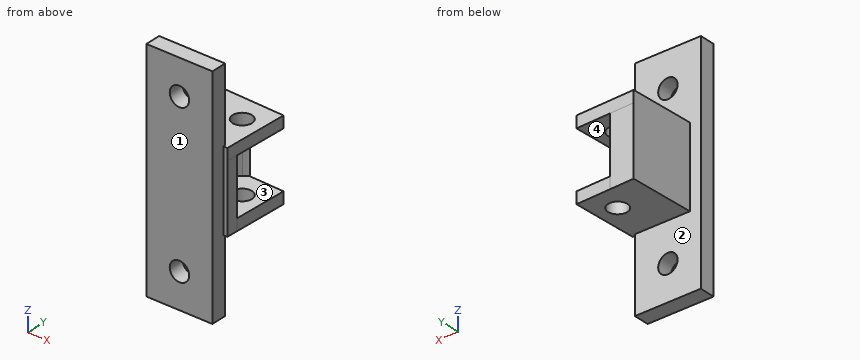
```python
from build123d import *

# Parameters (mm, degrees)
BOSS_EXTRUDE1_DEPTH = 22.352
BOSS_EXTRUDE3_START = -3.81
SKETCH2_R           = 3.175
BOSS_EXTRUDE3_DEPTH = 3.81
BOSS_EXTRUDE4_DEPTH = 3.81
CUT_EXTRUDE1_START  = -3.81
SKETCH6_R           = 3.175
CUT_EXTRUDE1_DEPTH  = 3.81
SKETCH7_W           = 21.59
SKETCH7_H           = 74.422
BOSS_EXTRUDE6_DEPTH = 5.08
SKETCH9_R           = 3.175
CUT_EXTRUDE2_DEPTH  = 6.35


with BuildPart() as part:
    # Sketch1 → Boss-Extrude1 (new body)
    with BuildSketch(Plane.XY):
        with BuildLine():
            ThreePointArc((-352.162161707, 117.383467749), (-351.384007065, 117.9545664), (-350.552048848, 118.44397813))
            Line((-350.552048848, 118.44397813), (-358.467972096, 118.728192663))
            Line((-358.467972096, 118.728192663), (-359.243555017, 97.126711503))
            Line((-359.243555017, 97.126711503), (-339.97264358, 96.434805718))
            Line((-339.97264358, 96.434805718), (-339.835936837, 100.242352338))
            Line((-339.835936837, 100.242352338), (-346.486451601, 100.481133449))
            ThreePointArc((-346.486451601, 100.481133449), (-349.816499797, 101.211177598), (-352.67617906, 103.067092457))
            ThreePointArc((-352.67617906, 103.067092457), (-355.663551295, 110.341766857), (-352.162161707, 117.383467749))
        make_face()
    extrude(amount=-BOSS_EXTRUDE1_DEPTH)

    # Sketch2 → Boss-Extrude3 (add)
    with BuildSketch(Plane(origin=(0, 0, -22.352), x_dir=(-1, 0, 0), z_dir=(0, 0, -1)).offset(BOSS_EXTRUDE3_START)):
        with BuildLine():
            ThreePointArc((346.486451601, 100.481133449), (355.434706729, 107.897354875), (350.552048848, 118.44397813))
            Line((350.552048848, 118.44397813), (339.197060659, 118.036286878))
            Line((339.197060659, 118.036286878), (339.835936837, 100.242352338))
            Line((339.835936837, 100.242352338), (346.486451601, 100.481133449))
        make_face()
        with Locations((346.144684744, 110)):
            Circle(SKETCH2_R, mode=Mode.SUBTRACT)
    extrude(amount=BOSS_EXTRUDE3_DEPTH)

    # Sketch3 → Boss-Extrude4 (add)
    with BuildSketch(Plane.XY):
        Polygon((-358.467972096, 118.728192663), (-359.243555017, 97.126711503), (-339.97264358, 96.434805718), (-339.197060659, 118.036286878), align=None)
    extrude(amount=BOSS_EXTRUDE4_DEPTH)

    # Sketch6 → Cut-Extrude1 (cut)
    with BuildSketch(Plane(origin=(0, 0, 0), x_dir=(-1, 0, 0), z_dir=(0, 0, -1)).offset(CUT_EXTRUDE1_START)):
        with Locations((346.144684744, 110)):
            Circle(SKETCH6_R)
    extrude(amount=CUT_EXTRUDE1_DEPTH, mode=Mode.SUBTRACT)

    # Sketch7 → Boss-Extrude6 (add)
    with BuildSketch(Plane(origin=(0, 97.126711503, 0), x_dir=(1, 0, 0), z_dir=(0, 1, 0))):
        with Locations((-352.044558269, 9.271)):
            Rectangle(SKETCH7_W, SKETCH7_H)
    extrude(amount=-BOSS_EXTRUDE6_DEPTH)

    # Sketch9 → Cut-Extrude2 (cut)
    with BuildSketch(Plane(origin=(0, 97.126711503, 0), x_dir=(1, 0, 0), z_dir=(0, 1, 0))):
        with Locations(Location((-352.044558269, -16.51, 0), (0, 0, 270))):
            Circle(SKETCH9_R)
        with Locations(Location((-352.044558269, 35.052, 0), (0, 0, 270))):
            Circle(SKETCH9_R)
    extrude(amount=-CUT_EXTRUDE2_DEPTH, mode=Mode.SUBTRACT)


solid = part.part
```
Build history of the part. All positions in model axes, mm. Face numbers are marked on the shaded views. Round coordinates to 2 decimals unless told otherwise and drop trailing zeros. Write each loop counter-clockwise with the first axis right and the second up, starting at its lowest first coordinate (ties: lowest second). Pieces come first, ordered by that corner, then holes. Notation, with made-up numbers: (53, -22.75) -> (109, -22.75) arc R21 ccw to (109, -3.75) -> close; hole circle Ø2 at (78, -18). An arc over 180 degrees is marked (long way). Put each result on its own line as item: value.
Item 1: Wall check: probe 1 along Z at (x, y) = (-350.5, 113.25); probe 2 along X at (y, z) = (94.2, 16.51); probe 3 along Y at (x, z) = (-358, 18.5). Give the ranges that are in metal, low to high. Write a range as from..to.
Here are the results:
probe 1: z = -22.35..-18.54, 0..3.81
probe 2: x = -362.84..-355.22, -348.87..-341.25
probe 3: y = 92.05..97.13
Item 2: Flat gauge pins, fed straight in: P1, Ø10, axis at x = -346.14, y = 110, coming from the +Z side; P2, Ø5, axis at x = -352.04, z = 16.51, coming from the -Y side; P3, Ø6, axis at x = -359, y = 109, coming from the -Z side; P4, Ø4, axis at x = -346, z = -17.5, coming from the +Y side. Where does each tip first touch, or does it go through?
Here are the results:
P1: stops at z = 3.81
P2: passes through
P3: stops at z = -22.35
P4: stops at y = 118.34
Item 3: Slice it at D-D, the plane y = 102. Give the cut face in (x, z), plus the area to 3 significant figures.
Here are the results:
outline: (-359.07, -22.35) -> (-339.77, -22.35) -> (-339.77, -18.54) -> (-351.31, -18.54) -> (-351.31, 0) -> (-339.77, 0) -> (-339.77, 3.81) -> (-359.07, 3.81) -> close
area: 291 mm^2
Item 4: Slice it at C-C, the plane y = 111. Give the cut face in (x, z).
Here are the results:
outline: (-358.75, -22.35) -> (-349.16, -22.35) -> (-349.16, -18.54) -> (-355.62, -18.54) -> (-355.62, 0) -> (-349.16, 0) -> (-349.16, 3.81) -> (-358.75, 3.81) -> close; (-343.13, -22.35) -> (-339.45, -22.35) -> (-339.45, -18.54) -> (-343.13, -18.54) -> close; (-343.13, 0) -> (-339.45, 0) -> (-339.45, 3.81) -> (-343.13, 3.81) -> close
Item 5: Slice it at A-A, the plane z = 2. Give the cut face in (x, y) (3 decimals).
Here are the results:
outline: (-362.84, 92.047) -> (-341.25, 92.047) -> (-341.25, 96.481) -> (-339.973, 96.435) -> (-339.197, 118.036) -> (-358.468, 118.728) -> (-359.244, 97.127) -> (-362.84, 97.127) -> close; hole circle Ø6.35 at (-346.145, 110)
Item 6: Two-plate mould, pull along Y, no slides. Class the marked faces 1, 2, 3 and 4: pulls with the +Y half, pulls with the -Y half, needs draft (parallel to the pull), parting line crosses it, or undercut.
Here are the results:
face 1: pulls with the -Y half
face 2: pulls with the +Y half
face 3: undercut
face 4: undercut
Item 7: Slice it at B-B, the plane z = 16.51. Give the cut face in (x, y), plus the area to 3 significant figures.
Here are the results:
outline: (-362.84, 92.05) -> (-355.22, 92.05) -> (-355.22, 97.13) -> (-362.84, 97.13) -> close; (-348.87, 92.05) -> (-341.25, 92.05) -> (-341.25, 97.13) -> (-348.87, 97.13) -> close
area: 77.4 mm^2
